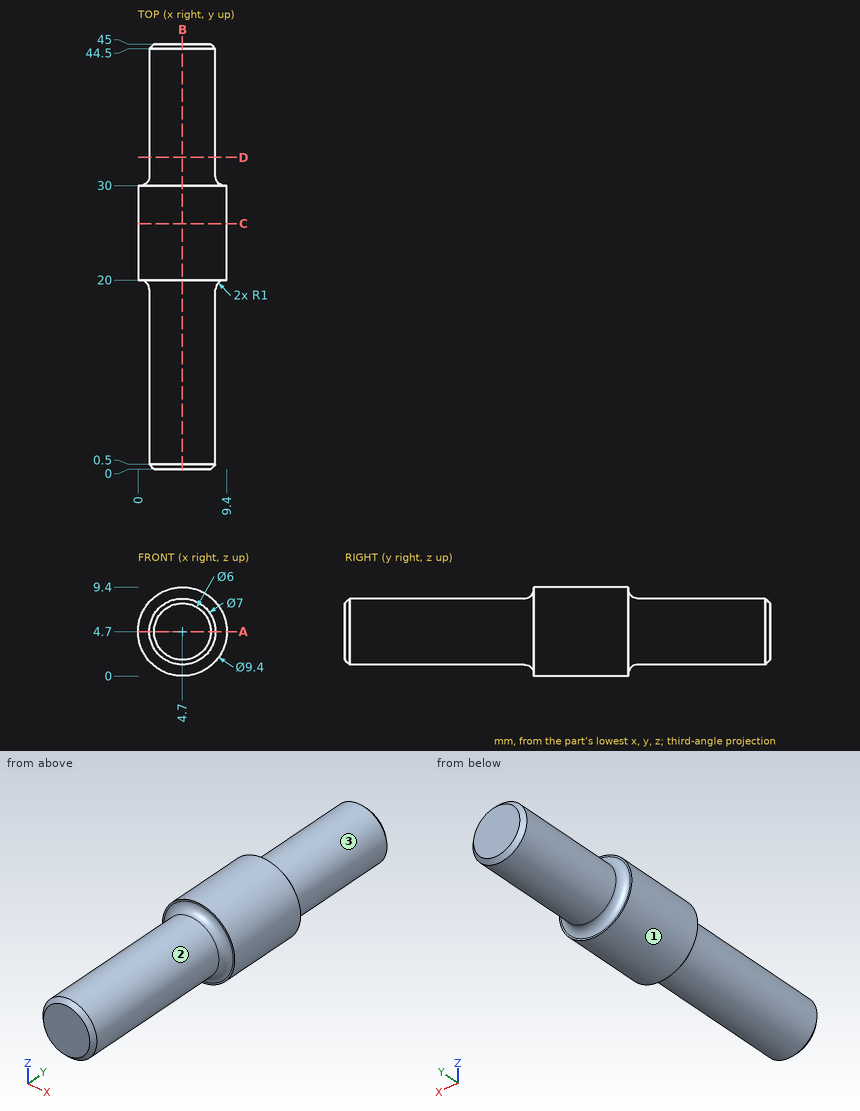
Study the drawing (mm; zero at the part's minimum x, y, z) and answer. A direction names the side the tool comes from. Give positions to 0.01 mm unless a question says otherwise; leave off trailing zeros. Order: outer loops, then holes, each group sorted by start corner. A loop starts at its lowest first (then second) coordinate and runs counter-clockwise, first axis right, second up. Notation, with made-up numbers: (58.5, 1) - (80.5, 1) arc R16 ccw to (80.5, 20) - close; hole circle Ø6 at (-14, 85.5). An arc over 180 degrees is marked (long way). Answer in a Markdown table with one row per item. Add a question column.
Q1. Given P1, Ø2, axis at x = 7, y = 21.5, coming from the -Z side, flat-ended and moving along its own axis, determine where the tip first touches the part or whether it passes through.
Q2. The part is cut by section A-A (z = 4.7). Determine the outline of the cut face in (x, y), then the cut area to 3 significant figures.
Q3. The part is cut by section B-B (x = 4.7). Determine the outline of the cut face in (y, z), then the cut area to 3 significant figures.
Q4. The part is cut by section C-C (y = 26). Determine the outline of the cut face in (x, z), then the cut area to 3 significant figures.
Q5. Which of the six approach directions +Z, -Z, +X, -X, +Y, -Y give full straight-line access (tool end or side, diameter ignored) to the marked faces 1, 2 and 3?
Q6. The part is cut by section D-D (y = 33). Determine the outline of the cut face in (x, z), then the cut area to 3 significant figures.
Q7. Find the intervals of material crossed by line 1 along Y through (x, z) = (3.5, 9); line 2 along X through (y, z) = (19, 7.25); line 3 along X through (y, z) = (5.5, 7.5), in increasing order. Write a range as [from, to].
Determined:
| question | item | result |
|---|---|---|
| 1 | P1 | stops at z = 0.18 |
| 2 | outline | (0, 20) - (0.2, 20) arc R1 cw to (1.2, 19) - (1.2, 0.5) - (1.7, 0) - (7.7, 0) - (8.2, 0.5) - (8.2, 19) arc R1 cw to (9.2, 20) - (9.4, 20) - (9.4, 30) - (9.2, 30) arc R1 cw to (8.2, 31) - (8.2, 44.5) - (7.7, 45) - (1.7, 45) - (1.2, 44.5) - (1.2, 31) arc R1 cw to (0.2, 30) - (0, 30) - close |
| 2 | area | 339 mm² |
| 3 | outline | (0, 1.7) - (0.5, 1.2) - (19, 1.2) arc R1 cw to (20, 0.2) - (20, 0) - (30, 0) - (30, 0.2) arc R1 cw to (31, 1.2) - (44.5, 1.2) - (45, 1.7) - (45, 7.7) - (44.5, 8.2) - (31, 8.2) arc R1 cw to (30, 9.2) - (30, 9.4) - (20, 9.4) - (20, 9.2) arc R1 cw to (19, 8.2) - (0.5, 8.2) - (0, 7.7) - close |
| 3 | area | 339 mm² |
| 4 | outline | circle Ø9.4 at (4.7, 4.7) |
| 4 | area | 69.4 mm² |
| 5 | face 1 | +Y, -Y |
| 5 | face 2 | -Y |
| 5 | face 3 | +Y |
| 6 | outline | circle Ø7 at (4.7, 4.7) |
| 6 | area | 38.5 mm² |
| 7 | line 1 | y = [20, 30] |
| 7 | line 2 | x = [2.3, 7.1] |
| 7 | line 3 | x = [2.6, 6.8] |
